Autodesk Inventor part; units mm, degrees
ref_plane "YZ Plane" through (0, 0, 0) normal (1, 0, 0) x (0, 1, 0)
ref_plane "XZ Plane" through (0, 0, 0) normal (0, 1, 0) x (-1, 0, 0)
ref_plane "XY Plane" through (0, 0, 0) normal (0, 0, 1) x (1, 0, 0)
sketch "Sketch1" plane through (0, 0, 0) normal (0, 1, 0) x (-1, 0, 0)
  line L0 (72.6415, 114.85) -> (-102.3585, 114.85)
  line L1 (-102.3585, 114.85) -> (-102.3585, -45.15)
  line L2 (-102.3585, -45.15) -> (72.6415, -45.15)
  line L3 (72.6415, -45.15) -> (72.6415, 114.85)
  line L4 (65.1415, 104.85) -> (-102.3585, 104.85)
  line L5 (-102.3585, 104.85) -> (-102.3585, -35.15)
  line L6 (-102.3585, -35.15) -> (65.1415, -35.15)
  line L7 (65.1415, -35.15) -> (65.1415, 104.85)
  line L8 (-102.3585, -35.15) -> (-89.8585, -35.15)
  line L9 (-89.8585, -35.15) -> (-89.8585, 104.85)
  line L10 (-89.8585, 104.85) -> (-102.3585, 104.85)
  line L11 (-102.3585, 104.85) -> (-102.3585, -35.15)
  point P0 (0, 0)
  dimension "d0" = 175
  dimension "d1" = 160
  dimension "d2" = 7.5
  dimension "d3" = 0
  dimension "d4" = 10
  dimension "d5" = 10
  dimension "d6" = 140
  dimension "d7" = 167.5
  dimension "d8" = 12.5
extrude "Extrusion1" add sketch "Sketch1" along normal blind 60 contours L3 L2 L1 L6 L7 L4 L0
sketch "Sketch2" plane through (-72.6415, 0, -45.15) normal (-1, 0, 0) x (0, 0, 1)
  line L0 (20, 52.5) -> (140, 52.5)
  line L1 (140, 52.5) -> (140, 25)
  line L2 (140, 25) -> (20, 25)
  line L3 (20, 25) -> (20, 52.5)
  line L4 (160, 0) -> (160, 60)
  line L5 (0, 0) -> (0, 60)
  line L6 (0, 60) -> (160, 60)
  line L7 (0, 0) -> (160, 0)
  point P0 (45.15, 0)
  dimension "d11" = 20
  dimension "d12" = 20
  dimension "d13" = 7.5
  dimension "d14" = 25
  dimension "d15" = 120
  dimension "d16" = 27.5
extrude "Extrusion2" cut sketch "Sketch2" against normal blind 60 contours L0 L1 L2 L3
sketch "Sketch3" plane through (0, 60, 0) normal (0, 1, 0) x (1, 0, 0)
  line L0 (-72.6415, -114.85) -> (102.3585, -114.85)
  line L1 (102.3585, 45.15) -> (-72.6415, 45.15)
  line L2 (-72.6415, -114.85) -> (102.3585, -114.85)
  line L3 (102.3585, -114.85) -> (102.3585, 45.15)
  line L4 (102.3585, 45.15) -> (-72.6415, 45.15)
  line L5 (-72.6415, 45.15) -> (-72.6415, -114.85)
  point P0 (0, 0)
extrude "Extrusion3" add sketch "Sketch3" along normal blind 7.5
sketch "Sketch4" plane through (0, 60, 0) normal (0, -1, 0) x (1, 0, 0)
  line L0 (-65.1415, 104.85) -> (102.3585, 104.85)
  line L1 (102.3585, -35.15) -> (-65.1415, -35.15)
  line L2 (102.3585, 104.85) -> (89.8585, 104.85)
  line L3 (89.8585, 104.85) -> (89.8585, -35.15)
  line L4 (89.8585, -35.15) -> (102.3585, -35.15)
  line L5 (102.3585, -35.15) -> (102.3585, 104.85)
  point P0 (0, 0)
  dimension "d21" = 12.5
extrude "Extrusion4" cut sketch "Sketch4" against normal blind 7.5
chamfer "Chamfer1" distance 30 angle 45 2 edges at (102.3585, 0, 109.85) (102.3585, 0, -40.15)
sketch "Sketch5" plane through (0, 67.5, 0) normal (0, 1, 0) x (1, 0, 0)
  line L0 (59.8585, -4.85) -> (29.8585, -4.85)
  line L1 (29.8585, -4.85) -> (29.8585, -29.85)
  line L2 (29.8585, -29.85) -> (59.8585, -29.85)
  line L3 (59.8585, -29.85) -> (59.8585, -4.85)
  line L4 (59.8585, -64.85) -> (29.8585, -64.85)
  line L5 (29.8585, -64.85) -> (29.8585, -39.85)
  line L6 (29.8585, -39.85) -> (59.8585, -39.85)
  line L7 (59.8585, -39.85) -> (59.8585, -64.85)
  line L8 (89.8585, -104.85) -> (89.8585, 35.15)
  line L9 (-72.6415, -114.85) -> (102.3585, -114.85)
  line L10 (102.3585, 45.15) -> (-72.6415, 45.15)
  point P0 (0, 0)
  dimension "d27" = 30
  dimension "d28" = 30
  dimension "d29" = 10
  dimension "d30" = 50
  dimension "d31" = 50
  dimension "d32" = 25
  dimension "d33" = 30
  dimension "d34" = 30
extrude "Extrusion5" cut sketch "Sketch5" against normal blind 7.5
sketch "Sketch6" plane through (0, 60, 0) normal (0, -1, 0) x (1, 0, 0)
  line L0 (64.8585, 69.85) -> (14.8585, 69.85)
  line L1 (14.8585, 69.85) -> (14.8585, -0.15)
  line L2 (14.8585, -0.15) -> (64.8585, -0.15)
  line L3 (64.8585, -0.15) -> (64.8585, 69.85)
  line L4 (59.8585, 64.85) -> (59.8585, 39.85)
  line L5 (29.8585, 39.85) -> (29.8585, 64.85)
  line L6 (29.8585, 64.85) -> (59.8585, 64.85)
  line L7 (59.8585, 4.85) -> (29.8585, 4.85)
  point P0 (0, 0)
  dimension "d37" = 5
  dimension "d38" = 15
  dimension "d39" = 5
  dimension "d40" = 5
extrude "Extrusion6" cut sketch "Sketch6" against normal blind 2.5
equation "\"d5\" = d4"
equation "\"d12\" = d11"
equation "\"d30\" = d31"
equation "\"d34\" = d33"
properties part number "Base-Motherboard"
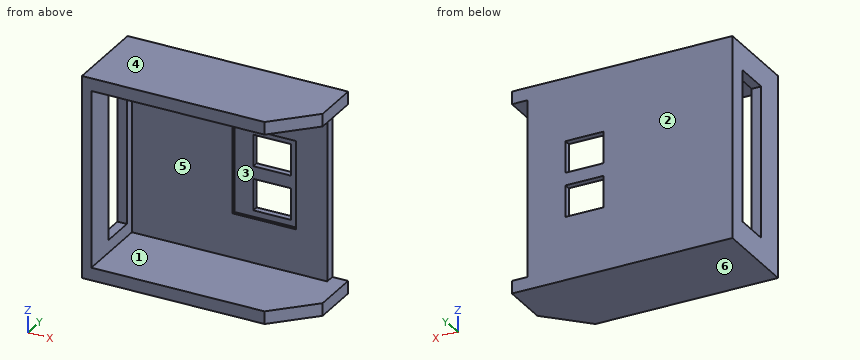
Check sheet for the modelled part. Datum: model origin and axes. Units: mm. Face numbers are marked on the shaded views. A direction names the side the tool comes from. Give positions to 0.01 mm unless a question says otherwise; leave off trailing zeros. Write each loop counter-clockwise with the first axis right and the second up, starting at its lowest first coordinate (ties: lowest second). Pieces come first, ordered by that corner, then holes. Notation, with made-up numbers: (37, -14.75) -> (89, -14.75) arc R19 ccw to (89, -1.75) -> close; hole circle Ø6 at (13.25, 88.25). An arc over 180 degrees is marked (long way). Use CSV: the item, a comma, the result in double quotes. Start each with the question number.
Q1. Release check for a two-part mould opening along Z. For the marked faces 4, 5 and 6 record: +Z half, -Z half, draft (parallel to the pull), parting line (faces both ways), or undercut.
Q2. Cross-section at B-B on z = 43.5. Enter the section's corners in (x, y), and give its area (3 significant figures).
Q3. Cross-section at D-D on z = 72. Enter the section's corners in (x, y).
Q4. Cross-section at A-A on y = 41. Enter the section's corners in (x, z), and give its area (3 significant figures).
Q5. Tool access check on the marked faces 1, 2 and 3. Record the directions out of +Z, -Z, +X, -X, +Y, -Y that give a thin tool (end or side, any length) a straight path to the whole face; none if there is none.
Q6. Scan lines: line 1 along Z through (x, y) = (-13, 22.5); line 2 along Y through (x, z) = (62.5, 63); line 3 along Y through (x, z) = (-20, 28.5). Record each from-to range of solid material in increasing order.
Q7. Depth check by flat-ended pin: P1, Ø3, axis at y = 16.5, z = 67, coming from the +X side; P2, Ø2.5, axis at y = 66, z = 21.5, coming from the +X side. Enter the tip coordinate at first touch or a pass-through.
Q8. Cross-section at C-C on x = -33.5. Enter the section's corners in (y, z).
Working result:
1,face 4,"+Z half"
1,face 5,"undercut"
1,face 6,"-Z half"
2,outline,"(-72.64, 0) -> (-65.14, 0) -> (-65.14, 25) -> (-72.64, 25) -> close; (-72.64, 52.5) -> (-65.14, 52.5) -> (-65.14, 60) -> (14.86, 60) -> (14.86, 62.5) -> (29.86, 62.5) -> (29.86, 67.5) -> (-72.64, 67.5) -> close; (59.86, 62.5) -> (64.86, 62.5) -> (64.86, 60) -> (89.86, 60) -> (89.86, 67.5) -> (59.86, 67.5) -> close"
2,area,"1,190 mm^2"
3,outline,"(-72.64, 0) -> (-65.14, 0) -> (-65.14, 25) -> (-72.64, 25) -> close; (-72.64, 52.5) -> (-65.14, 52.5) -> (-65.14, 60) -> (89.86, 60) -> (89.86, 67.5) -> (-72.64, 67.5) -> close"
4,outline,"(-72.64, -45.15) -> (102.36, -45.15) -> (102.36, -35.15) -> (-65.14, -35.15) -> (-65.14, -25.15) -> (-72.64, -25.15) -> close; (-72.64, 94.85) -> (-65.14, 94.85) -> (-65.14, 104.85) -> (102.36, 104.85) -> (102.36, 114.85) -> (-72.64, 114.85) -> close"
4,area,"3,650 mm^2"
5,face 1,"+X, -Y"
5,face 2,"+Z, -Z, +X, -X, +Y"
5,face 3,"-Y"
6,line 1,"z = -45.15 to -35.15, 104.85 to 114.85"
6,line 2,"y = 62.5 to 67.5"
6,line 3,"y = 60 to 67.5"
7,P1,"stops at x = -65.14"
7,P2,"stops at x = 89.86"
8,outline,"(0, -45.15) -> (67.5, -45.15) -> (67.5, 114.85) -> (0, 114.85) -> (0, 104.85) -> (60, 104.85) -> (60, -35.15) -> (0, -35.15) -> close"
